```python
from build123d import *

# Parameters (mm, degrees)
BOSS_EXTRU_1_DEPTH      = 20
ESQUISSE2_R             = 1.5
ENL_V_MAT_EXTRU_1_DEPTH = 20


with BuildPart() as part:
    # Esquisse1 → Boss.-Extru.1 (new body)
    with BuildSketch(Plane.XY):
        with BuildLine():
            Line((46, 12), (6, 12))
            ThreePointArc((6, 12), (0.456722805, 8.296100594), (1.757359313, 1.757359313))
            Line((1.757359313, 1.757359313), (3.171572875, 3.171572875))
            ThreePointArc((3.171572875, 3.171572875), (6, 10), (8.828427125, 3.171572875))
            Line((8.828427125, 3.171572875), (10.242640687, 1.757359313))
            ThreePointArc((10.242640687, 1.757359313), (11.997675746, 5.833010044), (10.472135955, 10))
            Line((10.472135955, 10), (32, 10))
            Line((32, 10), (32, 7.5))
            Line((32, 7.5), (38, 7.5))
            Line((38, 7.5), (38, 8.5))
            Line((38, 8.5), (33, 8.5))
            Line((33, 8.5), (33, 10))
            Line((33, 10), (41.527864045, 10))
            ThreePointArc((41.527864045, 10), (40.002324254, 5.833010044), (41.757359313, 1.757359313))
            Line((41.757359313, 1.757359313), (43.171572875, 3.171572875))
            ThreePointArc((43.171572875, 3.171572875), (46, 10), (48.828427125, 3.171572875))
            Line((48.828427125, 3.171572875), (50.242640687, 1.757359313))
            ThreePointArc((50.242640687, 1.757359313), (51.543277195, 8.296100594), (46, 12))
        make_face()
    extrude(amount=BOSS_EXTRU_1_DEPTH)

    # Esquisse2 → Enlèv. mat.-Extru.1 (cut)
    with BuildSketch(Plane(origin=(0, 12, 0), x_dir=(1, 0, 0), z_dir=(0, 1, 0))):
        with Locations(Location((26, -6, 0), (0, 0, 270))):
            Circle(ESQUISSE2_R)
        with Locations(Location((26, -14, 0), (0, 0, 270))):
            Circle(ESQUISSE2_R)
    extrude(amount=-ENL_V_MAT_EXTRU_1_DEPTH, mode=Mode.SUBTRACT)


solid = part.part
```
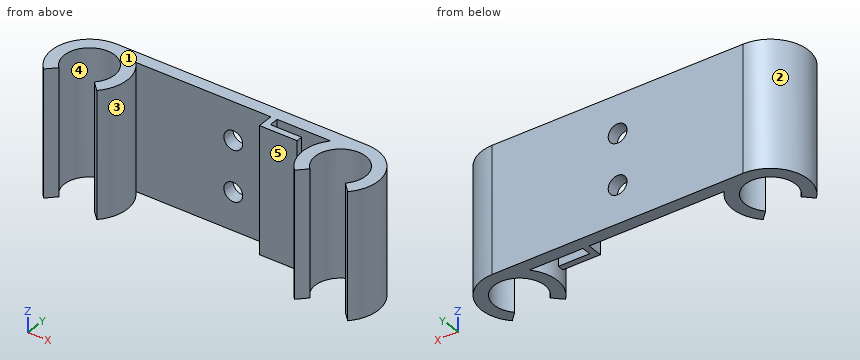
Work out the finished part from the listing and answer in its coordinate system (mm). Face numbers are marked on the shaded views. A direction names the side the tool comes from. Coordinates: 2 decimals unless noted, no trailing zeros. Order: outer loops, then holes, each group sorted by start corner. A loop starts at its lowest first (then second) coordinate and runs counter-clockwise, first axis right, second up. Notation, with made-up numbers: (32.5, 85.25) - (37.5, 85.25) arc R16 ccw to (37.5, 100.25) - close; hole circle Ø4 at (2, 72.25). An arc over 180 degrees is marked (long way). Answer as a JSON object with one key per item and string values.
1. Find section D-D on z = 9.5. Determine the outline of the cut face in (x, y).
Output values:
{"outline": "(1.76, 1.76) - (3.17, 3.17) arc R4 cw (long way) to (8.83, 3.17) - (10.24, 1.76) arc R6 ccw to (10.47, 10) - (32, 10) - (32, 7.5) - (38, 7.5) - (38, 8.5) - (33, 8.5) - (33, 10) - (41.53, 10) arc R6 ccw to (41.76, 1.76) - (43.17, 3.17) arc R4 cw (long way) to (48.83, 3.17) - (50.24, 1.76) arc R6 ccw to (46, 12) - (6, 12) arc R6 ccw to start"}
2. A tool of negligible diameter and unlimited length cuts with its end or side. For the marked faces 4 and 5, from which of +Z, -Z, +X, -X, +Y, -Y can it reach the whole face along a straight path? Write none if from no direction.
Output values:
{"face 4": "+Z, -Z", "face 5": "+Z, -Z, -Y"}
3. Consider line 1 (X direction, y = 6, z = 9.5); line 2 (X direction, y = 3.25, z = 9.75); line 3 (Y direction, x = 35.5, z = 6.75). Determine where each line is inside the solid, lowest interval first.
Output values:
{"line 1": "x = 0 to 2, 10 to 12, 40 to 42, 50 to 52", "line 2": "x = 0.67 to 3.1, 8.9 to 11.33, 40.67 to 43.1, 48.9 to 51.33", "line 3": "y = 7.5 to 8.5, 10 to 12"}
4. The mould has two halves that part along X. Classify the marked faces 1, 2 and 3: +X half, -X half, draft (parallel to the pull), parting line (faces both ways), or undercut.
Output values:
{"face 1": "draft", "face 2": "-X half", "face 3": "undercut"}
5. Find section C-C on x = 26. Determine the outline of the cut face in (y, z).
Output values:
{"outline": "(10, 0) - (12, 0) - (12, 4.5) - (10, 4.5) - close; (10, 7.5) - (12, 7.5) - (12, 12.5) - (10, 12.5) - close; (10, 15.5) - (12, 15.5) - (12, 20) - (10, 20) - close"}
6. Each of these flat-tipped pins is pushed along its axis until it touches: P1, Ø4, axis at y = 9, z = 14.5, coming from the +X side; P2, Ø1.1, axis at y = 8, z = 7, coming from the +X side; P3, Ø0.8, axis at y = 9.5, z = 12.5, coming from the +X side. Where does it stop, or does it pass through?
Output values:
{"P1": "stops at x = 51.92", "P2": "stops at x = 51.82", "P3": "stops at x = 51.14"}
7. Find section B-B on y = 6. Determine the outline of the cut face in (x, z).
Output values:
{"outline": "(0, 0) - (2, 0) - (2, 20) - (0, 20) - close; (10, 0) - (12, 0) - (12, 20) - (10, 20) - close; (40, 0) - (42, 0) - (42, 20) - (40, 20) - close; (50, 0) - (52, 0) - (52, 20) - (50, 20) - close"}
8. Find section A-A on z = 14. Determine the outline of the cut face in (x, y).
Output values:
{"outline": "(1.76, 1.76) - (3.17, 3.17) arc R4 cw (long way) to (8.83, 3.17) - (10.24, 1.76) arc R6 ccw to (10.47, 10) - (24.5, 10) - (24.5, 12) - (6, 12) arc R6 ccw to start; (27.5, 10) - (32, 10) - (32, 7.5) - (38, 7.5) - (38, 8.5) - (33, 8.5) - (33, 10) - (41.53, 10) arc R6 ccw to (41.76, 1.76) - (43.17, 3.17) arc R4 cw (long way) to (48.83, 3.17) - (50.24, 1.76) arc R6 ccw to (46, 12) - (27.5, 12) - close"}
